Source: CAD feature listing. Evaluate the final solid. Frame: model axes, mm. A direction names the side the tool comes from. Round coordinates to 2 decimals unless told otherwise and drop trailing zeros. Loops run counter-clockwise (first coordinate to the right, second up) from the corner with the lowest first, then second, coordinate; pieces in that order, holes last.
(1) Section A-A, the plane x = 362. Return the cut outline in (y, z), plus the area to 3 significant figures.
(2) Material intervals for probe 1 along Z at (x, y) = (261, -18); probe 2 along Y at (x, z) = (374.5, 19.5); probe 3 along X at (y, z) = (-15, 35), sorted ascending.
(3) Set-up query: faces 4 (the flat face through (19, -15, 36.195)), 5 (the flat face through (508, -9, 25)), 6 (the flat face through (4, -15, 22.225)). Return all of +Z, -Z, +X, -X, +Y, -Y with unobstructed straight access to the full face (end or side cutting, diameter ignored); none if empty.
(4) First-contact query: pin 1 Ø6.5 at (x, z) = (222, 28) entering from -Y; pin 2 Ø2.5 at (y, z) = (-13, 25.5) entering from -X; pin 3 Ø1.9 at (y, z) = (-16.5, 24.5) entering from -X. Flat tips, straight axial feed; report the tip coordinate or a pass-through.
(5) Mould query, pull axis Z, two halves, no side actions, for faces 1 (the flat face through (250, 0, 26)), 2 (the flat face through (250, -9, 0)), 3 (the flat face through (18, -15, 14.605)). Classes: pulls with the +Z half, pulls with the -Z half, needs draft (parallel to the pull), parting line crosses it, or undercut.
```python
from build123d import *

# Parameters (mm, degrees)
F0_W     = 508
F0_H     = 50.8
F1_DEPTH = 19.05
F3_DEPTH = 3.81
F5_DEPTH = 8.89


with BuildPart() as f1:
    # F0 (on Front) → F1 (new body)
    with BuildSketch(Plane.XZ):
        with Locations((254, 25.4)):
            Rectangle(F0_W, F0_H)
    extrude(amount=F1_DEPTH)

    # F2 (on face) → F3 (cut)
    with BuildSketch(Plane.XZ.offset(19.05)):
        with BuildLine():
            Line((492.125, 32.004), (27.94, 32.004))
            Line((27.94, 32.004), (27.94, 33.02))
            ThreePointArc((27.94, 33.02), (27.010064, 35.265064), (24.765, 36.195))
            Line((24.765, 36.195), (12.065, 36.195))
            ThreePointArc((12.065, 36.195), (9.819936, 35.265064), (8.89, 33.02))
            Line((8.89, 33.02), (8.89, 28.575))
            Line((8.89, 28.575), (0, 28.575))
            Line((0, 28.575), (0, 22.225))
            Line((0, 22.225), (8.89, 22.225))
            Line((8.89, 22.225), (8.89, 17.78))
            ThreePointArc((8.89, 17.78), (9.819936, 15.534936), (12.065, 14.605))
            Line((12.065, 14.605), (24.765, 14.605))
            ThreePointArc((24.765, 14.605), (27.010064, 15.534936), (27.94, 17.78))
            Line((27.94, 17.78), (27.94, 18.796))
            Line((27.94, 18.796), (492.125, 18.796))
            ThreePointArc((492.125, 18.796), (494.370064, 19.725936), (495.3, 21.971))
            Line((495.3, 21.971), (495.3, 28.829))
            ThreePointArc((495.3, 28.829), (494.370064, 31.074064), (492.125, 32.004))
        make_face()
    extrude(amount=-F3_DEPTH, mode=Mode.SUBTRACT)

    # F4 (on face) → F5 (cut)
    with BuildSketch(Plane.XZ.offset(19.05)):
        with BuildLine():
            Line((12.065, 14.605), (24.765, 14.605))
            ThreePointArc((24.765, 14.605), (27.010064, 15.534936), (27.94, 17.78))
            Line((27.94, 17.78), (27.94, 33.02))
            ThreePointArc((27.94, 33.02), (27.010064, 35.265064), (24.765, 36.195))
            Line((24.765, 36.195), (12.065, 36.195))
            ThreePointArc((12.065, 36.195), (9.819936, 35.265064), (8.89, 33.02))
            Line((8.89, 33.02), (8.89, 28.575))
            Line((8.89, 28.575), (-2.839666, 28.575))
            ThreePointArc((-2.839666, 28.575), (-5.08473, 27.645064), (-6.014666, 25.4))
            ThreePointArc((-6.014666, 25.4), (-5.08473, 23.154936), (-2.839666, 22.225))
            Line((-2.839666, 22.225), (8.89, 22.225))
            Line((8.89, 22.225), (8.89, 17.78))
            ThreePointArc((8.89, 17.78), (9.819936, 15.534936), (12.065, 14.605))
        make_face()
    extrude(amount=-F5_DEPTH, mode=Mode.SUBTRACT)


solid = f1.part
```
Output values:
1. outline: (-19.05, 0) - (0, 0) - (0, 50.8) - (-19.05, 50.8) - (-19.05, 32) - (-15.24, 32) - (-15.24, 18.8) - (-19.05, 18.8) - close
1. area: 917 mm2
2. probe 1: z = 0 to 18.8, 32 to 50.8
2. probe 2: y = -15.24 to 0
2. probe 3: x = 0 to 9.58, 27.25 to 508
3. face 4: -Y
3. face 5: +Z, -Z, +X, +Y, -Y
3. face 6: -X, -Y
4. pin 1: stops at y = -15.24
4. pin 2: stops at x = 27.94
4. pin 3: stops at x = 495.3
5. face 1: needs draft
5. face 2: pulls with the -Z half
5. face 3: undercut
